Source: CAD feature listing. Evaluate the final solid. Frame: model axes, mm. A direction names the side the tool comes from. Round coordinates to 2 decimals unless told otherwise and drop trailing zeros. Write each loop counter-clockwise with the first axis right and the second up, starting at its lowest first coordinate (ties: lowest second). Pieces come first, ordered by that corner, then holes. Notation, with made-up numbers: M 33.25,-34.5 L 71.25,-34.5 A13 ccw 71.25,-13.5 Z; hole C -35,-34.75 d2. An arc over 180 degrees is marked long. Use a Markdown table: item, result.
```python
from build123d import *

# Parameters (mm, degrees)
F0_R     = 34.544
F1_DEPTH = 6.35
F0_R_2   = 40.64
F2_DEPTH = 12.7


with BuildPart() as f1:
    # F0 (on Top) → F1 (new body)
    with BuildSketch(Plane.XY):
        Circle(F0_R)
        with BuildLine():
            ThreePointArc((-31.076682867, -5.1222844495), (-24.0138448298, 20.3797269974), (0, 31.496))
            Line((0, 31.496), (0, 10.922))
            Line((0, 10.922), (-10.414, 10.922))
            Line((-10.414, 10.922), (-10.5108203487, 18.2749385662))
            ThreePointArc((-10.5108203487, 18.2749385662), (-16.9420488689, 12.5466212234), (-20.5458211965, 4.7244))
            Line((-20.5458211965, 4.7244), (0, 4.7244))
            Line((0, 4.7244), (0, -31.496))
            ThreePointArc((0, -31.496), (-18.2512319231, -25.6688634203), (-29.7490715955, -10.3436335592))
            Line((-29.7490715955, -10.3436335592), (-18.3700835271, -10.3436335592))
            ThreePointArc((-18.3700835271, -10.3436335592), (-14.9357796661, -14.8786158552), (-10.414, -18.3302844495))
            Line((-10.414, -18.3302844495), (-10.414, -5.1222844495))
            Line((-10.414, -5.1222844495), (-31.076682867, -5.1222844495))
        make_face(mode=Mode.SUBTRACT)
        with BuildLine():
            ThreePointArc((19.8204750869, -24.4774750195), (15.3939322044, -27.477715831), (10.523637749, -29.6858731475))
            Line((10.523637749, -29.6858731475), (10.523637749, -13.6838731475))
            Line((10.523637749, -13.6838731475), (19.8204750869, -24.4774750195))
        make_face(mode=Mode.SUBTRACT)
        with BuildLine():
            ThreePointArc((31.0882471472, -5.0516240273), (29.9760430145, -9.6661709684), (28.1829993455, -14.0611722091))
            ThreePointArc((28.1829993455, -14.0611722091), (27.753918864, -14.8901982421), (27.3004586922, -15.7061443772))
            Line((27.3004586922, -15.7061443772), (17.8802471472, -5.0516240273))
            Line((17.8802471472, -5.0516240273), (31.0882471472, -5.0516240273))
        make_face(mode=Mode.SUBTRACT)
        with BuildLine():
            ThreePointArc((10.3465438025, 18.3684445543), (16.8012840648, 12.7345034365), (20.4811438025, 4.9973465502))
            Line((20.4811438025, 4.9973465502), (10.3465438025, 4.9973465502))
            Line((10.3465438025, 4.9973465502), (10.3465438025, 18.3684445543))
        make_face(mode=Mode.SUBTRACT)
    extrude(amount=F1_DEPTH)

    # F0 (on Top) → F2 (join)
    with BuildSketch(Plane.XY):
        Circle(F0_R_2)
        Circle(F0_R, mode=Mode.SUBTRACT)
        with BuildLine():
            Line((0, 10.922), (0, 31.496))
            ThreePointArc((0, 31.496), (-24.0138448298, 20.3797269974), (-31.076682867, -5.1222844495))
            Line((-31.076682867, -5.1222844495), (-10.414, -5.1222844495))
            Line((-10.414, -5.1222844495), (-10.414, -18.3302844495))
            ThreePointArc((-10.414, -18.3302844495), (-14.9357796661, -14.8786158552), (-18.3700835271, -10.3436335592))
            Line((-18.3700835271, -10.3436335592), (-29.7490715955, -10.3436335592))
            ThreePointArc((-29.7490715955, -10.3436335592), (-18.2512319231, -25.6688634203), (0, -31.496))
            Line((0, -31.496), (0, 4.7244))
            Line((0, 4.7244), (-20.5458211965, 4.7244))
            ThreePointArc((-20.5458211965, 4.7244), (-16.9420488689, 12.5466212234), (-10.5108203487, 18.2749385662))
            Line((-10.5108203487, 18.2749385662), (-10.414, 10.922))
            Line((-10.414, 10.922), (0, 10.922))
        make_face()
        with BuildLine():
            Line((10.3465438025, 4.9973465502), (20.4811438025, 4.9973465502))
            ThreePointArc((20.4811438025, 4.9973465502), (16.8012840648, 12.7345034365), (10.3465438025, 18.3684445543))
            Line((10.3465438025, 18.3684445543), (10.3465438025, 4.9973465502))
        make_face()
        with BuildLine():
            Line((10.523637749, -13.6838731475), (10.523637749, -29.6858731475))
            ThreePointArc((10.523637749, -29.6858731475), (15.3939322044, -27.477715831), (19.8204750869, -24.4774750195))
            Line((19.8204750869, -24.4774750195), (10.523637749, -13.6838731475))
        make_face()
        with BuildLine():
            ThreePointArc((27.3004586922, -15.7061443772), (27.753918864, -14.8901982421), (28.1829993455, -14.0611722091))
            ThreePointArc((28.1829993455, -14.0611722091), (29.9760430145, -9.6661709684), (31.0882471472, -5.0516240273))
            Line((31.0882471472, -5.0516240273), (17.8802471472, -5.0516240273))
            Line((17.8802471472, -5.0516240273), (27.3004586922, -15.7061443772))
        make_face()
    extrude(amount=F2_DEPTH)


solid = f1.part
```
Q1. Section D-D on x = -27. Return loops of the section in (y, z), plus the area to 3 significant figures.
Results are:
| item | result |
|---|---|
| outline | M -30.37,0 L 30.37,0 L 30.37,12.7 L 21.55,12.7 L 21.55,6.35 L 16.22,6.35 L 16.22,12.7 L -5.12,12.7 L -5.12,6.35 L -10.34,6.35 L -10.34,12.7 L -16.22,12.7 L -16.22,6.35 L -21.55,6.35 L -21.55,12.7 L -30.37,12.7 Z |
| area | 671 mm^2 |
Q2. Line query: L1, parallel to Y at x = 26.5, z = 7.25; L2, parallel to Y at x = 23, z = 6.75; L3, parallel to Y at x = -13.5, z = 11.5. Output: solid intervals per line, ascending.
Results are:
| item | result |
|---|---|
| L1 | -30.81 to -22.16, -14.8 to -5.05, 22.16 to 30.81 |
| L2 | -33.51 to -25.77, -10.84 to -5.05, 25.77 to 33.51 |
| L3 | -38.33 to -31.8, -28.46 to -16.19, -5.12 to 4.72, 16.19 to 28.46, 31.8 to 38.33 |
Q3. Mould query, pull axis Y, two halves, no side actions, for faces 1 (the cylindrical face through (-5.291, 40.294, 6.261)), 2 (the flat face through (-12, 0, 12.7)), 3 (the flat face through (-5, 10.922, 9)). Classes: +Y half, -Y half, draft (parallel to the pull), parting line (faces both ways), or undercut.
Results are:
| item | result |
|---|---|
| face 1 | parting line |
| face 2 | draft |
| face 3 | undercut |
Q4. Section B-B on x = -15. Return loops of the section in (y, z).
Results are:
| item | result |
|---|---|
| outline | M -37.77,0 L 37.77,0 L 37.77,12.7 L 31.12,12.7 L 31.12,6.35 L 27.69,6.35 L 27.69,12.7 L 14.81,12.7 L 14.81,6.35 L 4.72,6.35 L 4.72,12.7 L -5.12,12.7 L -5.12,6.35 L -14.81,6.35 L -14.81,12.7 L -27.69,12.7 L -27.69,6.35 L -31.12,6.35 L -31.12,12.7 L -37.77,12.7 Z |
Q5. Reachability of faces 4 (the flat face through (10.347, 12, 9)), 5 (the flat face through (14, 10, 12.7)) from +Z, -Z, +X, -X, +Y, -Y: full face, straight path, thin tool, end or side. Return the list, or none.
Results are:
| item | result |
|---|---|
| face 4 | +Z |
| face 5 | +Z, +X, -X, +Y, -Y |
Q6. Section A-A on y = 0. Return loops of the section in (x, z), plus the area to 3 significant figures.
Results are:
| item | result |
|---|---|
| outline | M -40.64,0 L 40.64,0 L 40.64,12.7 L 34.54,12.7 L 34.54,6.35 L 0,6.35 L 0,12.7 L -31.5,12.7 L -31.5,6.35 L -34.54,6.35 L -34.54,12.7 L -40.64,12.7 Z |
| area | 794 mm^2 |
Q7. First-contact query: pin 1 Ø1.9 at (x, z) = (-22, 10) entering from +Y; pin 2 Ø1.9 at (y, z) = (13.5, 10.5) entering from -X; pin 3 Ø6 at (x, z) = (21, 1.5) entering from +Y; pin 4 Ø12 at (x, y) = (0.5, 22.5) entering from +Z. Flat tips, straight axial feed; report the tip coordinate or a pass-through.
Results are:
| item | result |
|---|---|
| pin 1 | y = 34.76 |
| pin 2 | x = -38.65 |
| pin 3 | y = 36.44 |
| pin 4 | z = 12.7 |
Q8. Section C-C on z = 3.75. Return loops of the section in (x, y), plus the area to 3 significant figures.
Results are:
| item | result |
|---|---|
| outline | C 0,0 d81.28 |
| area | 5,190 mm^2 |
